```python
from build123d import *

# Parameters (mm, degrees)
SKETCH2_W          = 100
SKETCH2_H          = 120
CUT_EXTRUDE1_DEPTH = 82
SKETCH4_R          = 50
CUT_EXTRUDE2_DEPTH = 20


with BuildPart() as part:
    # Sketch1 → Revolve1 (revolve)
    with BuildSketch(Plane(origin=(0, 0, 0), x_dir=(1, 0, 0), z_dir=(0, 1, 0)), mode=Mode.PRIVATE) as revolve1_sk:
        with BuildLine():
            Line((0, 0), (-150, 0))
            Line((-150, 0), (-150, 60))
            Line((-150, 60), (3.289990225, 49.891642229))
            ThreePointArc((3.289990225, 49.891642229), (36.499996652, 34.172360825), (50, 0))
            Line((50, 0), (0, 0))
        make_face()
    revolve(revolve1_sk.sketch.rotate(Axis((0, 0, 0), (-1, 0, 0)), 180), axis=Axis((0, 0, 0), (-1, 0, 0)))

    # Sketch2 → Cut-Extrude1 (cut)
    with BuildSketch(Plane(origin=(0, 0, 0), x_dir=(1, 0, 0), z_dir=(0, 1, 0))):
        with Locations((3.289990225, 0)):
            Rectangle(SKETCH2_W, SKETCH2_H)
    extrude(amount=CUT_EXTRUDE1_DEPTH, mode=Mode.SUBTRACT)

    # Sketch3 → Revolve2 (revolve)
    with BuildSketch(Plane(origin=(0, 0, 0), x_dir=(1, 0, 0), z_dir=(0, 1, 0))):
        with BuildLine():
            Line((-35, 0), (35, 0))
            ThreePointArc((35, 0), (0, 35), (-35, 0))
        make_face()
    revolve(axis=Axis((-35, 0, 0), (1, 0, 0)))

    # Sketch4 → Cut-Extrude2 (cut)
    with BuildSketch(Plane.ZY.offset(150)):
        Circle(SKETCH4_R)
    extrude(amount=-CUT_EXTRUDE2_DEPTH, mode=Mode.SUBTRACT)


solid = part.part
```
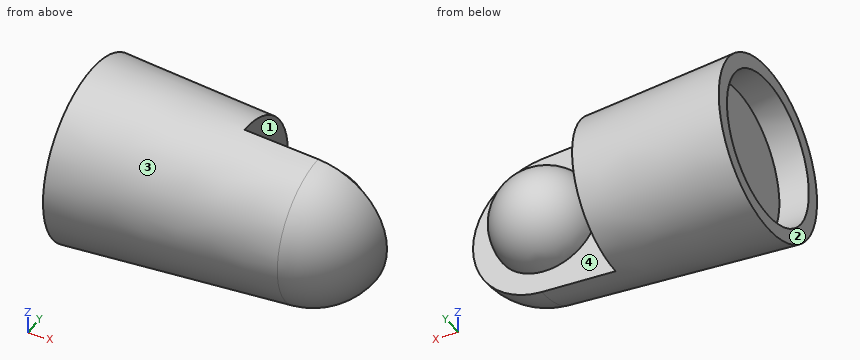
Verification items for the finished model (mm, model axes). Face numbers are marked on the shaded views. Round coordinates to 2 decimals unless told otherwise and drop trailing zeros. Order: outer loops, then holes, each group sorted by start corner. A loop starts at its lowest first (then second) coordinate and runs counter-clockwise, first axis right, second up.
1) Material ranges on line 1 (Y direction, x = -139.25, z = 0); line 2 (Y direction, x = -144.75, z = 0); line 3 (X direction, y = 24.5, z = -15.5), recorded low to high.
Geometry says:
line 1: y = -59.29 to -50, 50 to 59.29
line 2: y = -59.65 to -50, 50 to 59.65
line 3: x = -130 to -46.71, -19.61 to 19.61
2) Depth check by flat-ended pin: pin 1 (1 mm diameter, centred on x = -48.5, z = -30.5, fed in from -Y); pin 2 (8 mm diameter, centred on x = 26.5, z = 33.5, fed in from +Y); pin 3 (12 mm diameter, centred on x = -94, z = -14.5, fed in from +Y); pin 4 (10 mm diameter, centred on x = -25, y = 33, fed in from -Z) (3 decimals). Enter the tip coordinate at first touch or a pass-through.
Geometry says:
pin 1: stops at y = -44.07
pin 2: stops at y = 0
pin 3: stops at y = 55.74
pin 4: passes through
3) Cross-section at A-A, the plane z = 0. Record the cut outline in (x, y), plus the area to 3 significant figures.
Geometry says:
outline: (-150, -60) - (3.29, -49.89) arc R50 ccw to (50, 0) - (35, 0) arc R35 ccw to (-35, 0) - (-46.71, 0) - (-46.71, 53.19) - (-150, 60) - (-150, 50) - (-130, 50) - (-130, -50) - (-150, -50) - close
area: 16,000 mm2
4) Cross-section at C-C, the plane x = -17. Record the cut outline in (y, z).
Geometry says:
outline: (0, -51.23) - (0, -30.59) arc R30.59 ccw to (0, 30.59) - (0, 51.23) arc R51.23 ccw to start
5) Draft check along X on the marked faces 1, 2, 3 and 4. Enter one of: +X half, -X half, draft (parallel to the pull), parting line (faces both ways), or undercut.
Geometry says:
face 1: undercut
face 2: -X half
face 3: +X half
face 4: undercut
6) Cross-section at B-B, the plane x = -108.5. Record the cut outline in (y, z).
Geometry says:
outline: circle Ø114.53 at (0, 0)
